```python
from build123d import *

# Parameters (mm, degrees)
F0_R     = 31.75
F1_DEPTH = 63.5
F2_R     = 5.08
F4_D     = 6.7564


with BuildPart() as f1:
    # F0 (on Front) → F1 (new body)
    with BuildSketch(Plane.XZ):
        with Locations((-34.2211462557, 0)):
            Circle(F0_R)
    extrude(amount=F1_DEPTH)

    # F2
    f2_edges = [f1.edges().sort_by_distance(p)[0] for p in [
        (-2.471146, -31.75, 0),
        (-65.971146, 0, 0),
        (-65.971146, -63.5, 0),
    ]]
    fillet(f2_edges, radius=F2_R)

    # F4 (through all)
    with Locations(Plane.XZ.offset(63.5)):
        with Locations((-24.5181079954, 5.975802429), (-37.0556861162, 14.9742206559), (-48.9838346839, -9.0467510745), (-37.0556861162, -17.8351700306)):
            Hole(F4_D / 2)


solid = f1.part
```
The model under review builds one solid part; all positions refer to its coordinate system, in mm. Round coordinates to 2 decimals unless told otherwise and drop trailing zeros. Write each loop counter-clockwise with the first axis right and the second up, starting at its lowest first coordinate (ties: lowest second). Pieces come first, ordered by that corner, then holes. Notation, with made-up numbers: (51.25, 48) -> (87.25, 48) arc R28 ccw to (87.25, 84) -> close; hole circle Ø1 at (60.5, 50). An arc over 180 degrees is marked (long way). Use CSV: the item, a comma, the result in double quotes.
Q1. Consider section A-A (y = -6.5). Give the boundary of the cut face in (x, z), then the cut area to 3 significant figures.
Checks:
outline,"circle Ø63.5 at (-34.22, 0); hole circle Ø6.76 at (-48.98, -9.05); hole circle Ø6.76 at (-37.06, -17.84); hole circle Ø6.76 at (-37.06, 14.97); hole circle Ø6.76 at (-24.52, 5.98)"
area,"3,020 mm²"
Q2. For pin 1 Ø11 at (x, z) = (-24.52, 5.98) entering from +Y; pin 2 Ø6 at (x, z) = (-37.06, -17.84) entering from +Y; pin 3 Ø3 at (x, y) = (-40, -40.5) entering from -Z; pin 4 Ø6 at (y, z) = (-20, 4) entering from +X, all flat-tipped, find the tip position at first contact; note any pin that passes through.
Checks:
pin 1,"y = 0"
pin 2,"through"
pin 3,"z = -31.46"
pin 4,"x = -2.49"
Q3. To check wall thickness, follow probe 1 along Z at (x, y) = (-46, -51); probe 2 along Z at (x, y) = (-21.5, -54); probe 3 along X at (y, z) = (-24.5, -6). State the ranges of each line that lie inside material, in increasing order. Write a range as [from, to].
Checks:
probe 1,"[-29.48, -10.63], [-7.46, 29.48]"
probe 2,"[-29.09, 4.46], [7.49, 29.09]"
probe 3,"[-65.4, -50.44], [-47.52, -3.04]"
Q4. Mouldability with a two-part tool opening along X and no side actions: class faces 1 (the cylindrical face through (-34.57, -31.31, -15.55)), 2 (the cylindrical face through (-59.417, -31.377, -19.319)), 3 (the flat face through (-35, -63.5, 0)), 4 (the cylindrical face through (-27.64, -31.31, 4.68)) as released by +X, released by -X, zero draft, split by the parting line, or undercut.
Checks:
face 1,"undercut"
face 2,"split by the parting line"
face 3,"zero draft"
face 4,"undercut"
